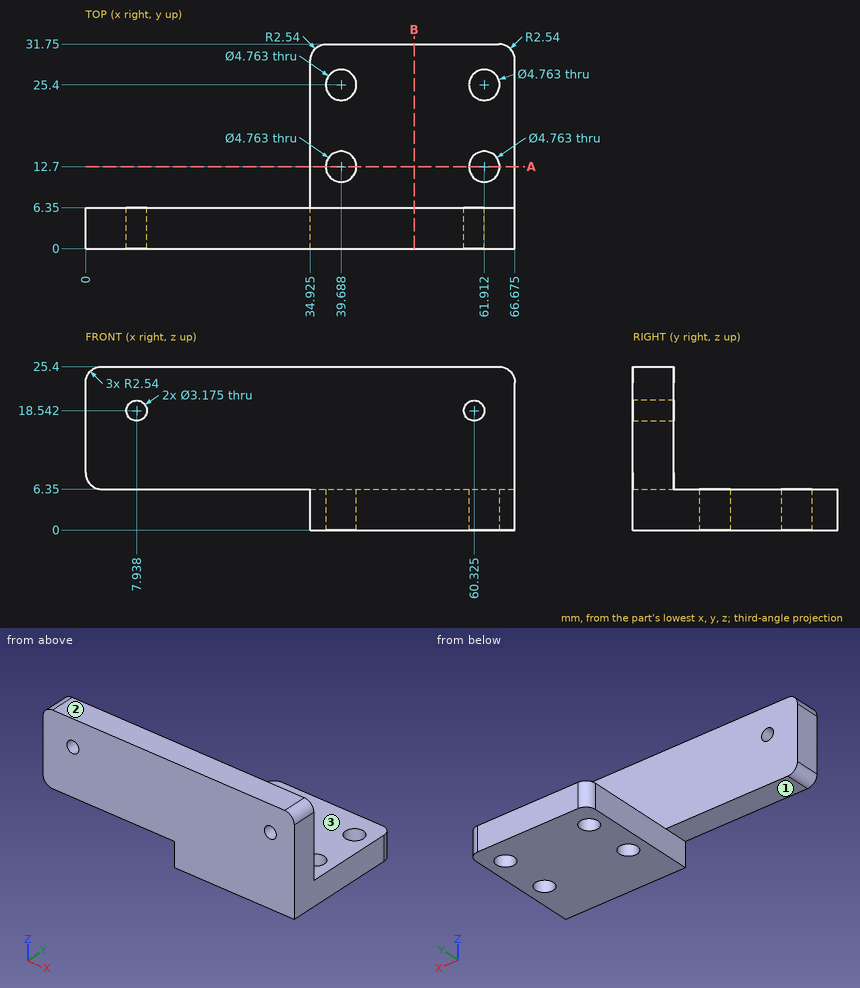
Here's the drawing with two shaded views (mm, measured from the low corner). I have some questions. A direction names the side the tool comes from. Give positions to 0.01 mm unless a question says otherwise; leave off trailing zeros. Loops run counter-clockwise (first coordinate to the right, second up) from the corner with the lowest first, then second, coordinate; pieces in that order, holes last. Notation, with made-up numbers: M 65.5,54 L 89.5,54 A19 cw 89.5,60 Z; hole C -35.5,-18 d10. An arc over 180 degrees is marked long. One line per item, written item: value. Start each with the question number.
1) On a 3-axis mill with a long thin cutter (end or side, diameter ignored), from which of +Z, -Z, +X, -X, +Y, -Y can I reach the whole of each face in a straight line? I mean the marked faces 1, 2 and 3. Say none if no direction works.
2) If we section it at B-B, the plane x = 51: Write out the boundary of the cut face in (y, z).
3) If we section it at A-A, the plane y = 12.7: Give the number of separate pieces and of enclosed holes in the cut face, and give its area (3 significant figures).
4) If I drill on line 1 (X direction, y = 12, z = 1.25) (1 decimal); line 2 (Y direction, x = 5, z = 15.5), over which ranges is the centre line in solid material (lowest first)? Write a range as [from, to].
5) I'm going to push flat-ended pins straight in: pin 1 (12 mm diameter, centred on x = 58, z = 19.5, fed in from +Y); pin 2 (4 mm diameter, centred on x = 7.94, z = 18.54, fed in from -Y); pin 3 (7.5 mm diameter, centred on x = 61.91, y = 25.4, fed in from +Z); pin 4 (1.9 mm diameter, centred on y = 19.5, z = 4, fed in from -X) (1 decimal). Where does each tip first touch, or does it pass through?
Completed:
1. face 1: -Z, -X, +Y, -Y
1. face 2: +Z, +X, -X, +Y, -Y
1. face 3: +Z, +X, -X, +Y
2. outline: M 0,0 L 31.75,0 L 31.75,6.35 L 6.35,6.35 L 6.35,25.4 L 0,25.4 Z
3. separate pieces: 3
3. enclosed holes: 0
3. area: 141 mm^2
4. line 1: x = [34.9, 37.4], [42, 59.6], [64.2, 66.7]
4. line 2: y = [0, 6.35]
5. pin 1: stops at y = 6.35
5. pin 2: stops at y = 0
5. pin 3: stops at z = 6.35
5. pin 4: stops at x = 34.9
